from build123d import *
from build123d.topology import SkipClean

# Parameters (mm, degrees)
SKETCH1_W            = 10
SKETCH1_H            = 10
BOSS_EXTRUDE1_DEPTH  = 4.9
CHAMFER1_SIZE        = 1
BOSS_EXTRUDE2_DEPTH  = 16
BOSS_EXTRUDE3_DEPTH  = 10
BOSS_EXTRUDE4_DEPTH  = 13
CHAMFER2_SIZE        = 12
BOSS_EXTRUDE5_DEPTH  = 30
CUT_EXTRUDE2_REACH   = 128.798
CUT_EXTRUDE1_START   = -15
CUT_EXTRUDE1_DEPTH   = 15
M3_CLEARANCE_HOLE1_D = 3.6
SKETCH11_W           = 1.8
SKETCH11_H           = 4.9
CHAMFER3_SIZE        = 9
CHAMFER3_SIZE_2      = 7.926193673
SKETCH14_R           = 1.8
BOSS_EXTRUDE6_DEPTH  = 12
M3_CLEARANCE_HOLE3_D = 3.6
SKETCH19_W           = 25
SKETCH19_H           = 20
CUT_EXTRUDE3_DEPTH   = 3.062116


# Read off the part's stored shape, not the designer's step: Cut-Extrude1
# Some blends are built 0.0001 mm under size
with BuildPart() as part:
    # Sketch1 → Boss-Extrude1 (new body)
    with BuildSketch(Plane(origin=(0, 0, 0), x_dir=(1, 0, 0), z_dir=(0, 1, 0))):
        with Locations((-5, 5)):
            Rectangle(SKETCH1_W, SKETCH1_H)
    extrude(amount=BOSS_EXTRUDE1_DEPTH)

    # Chamfer1
    chamfer1_edges = [part.edges().sort_by_distance(p)[0] for p in [
        (-10, 0, -5),
    ]]
    chamfer(chamfer1_edges, length=CHAMFER1_SIZE)

    # Sketch2 → Boss-Extrude2 (add)
    with BuildSketch(Plane(origin=(0, 0, -10), x_dir=(-1, 0, 0), z_dir=(0, 0, -1))):
        Polygon((-49.9, -10.1), (-48.419662682, -10.1), (-46.146212445, -7.037883957), (1.467233005, 0), (9, 0), (10, 1), (10, 4.9), (0, 4.9), (-45.9, -1.884614526), (-45.9, 4.9), (-95.9, 4.9), (-95.9, 1.9), (-49.9, 1.9), align=None)
    extrude(amount=BOSS_EXTRUDE2_DEPTH)

    # Sketch2<4> → Boss-Extrude3 (add)
    with BuildSketch(Plane(origin=(0, 0, -10), x_dir=(-1, 0, 0), z_dir=(0, 0, -1))):
        Polygon((-49.9, -10.1), (-48.419662682, -10.1), (-46.146212445, -7.037883957), (1.467233005, 0), (0, 0), (0, 4.9), (-45.9, -1.884614526), (-45.9, 4.9), (-95.9, 4.9), (-95.9, 1.9), (-49.9, 1.9), align=None)
    extrude(amount=-BOSS_EXTRUDE3_DEPTH)

    # Sketch3 → Boss-Extrude4 (add)
    with BuildSketch(Plane(origin=(0, 0, -26), x_dir=(-1, 0, 0), z_dir=(0, 0, -1))):
        Polygon((-95.9, 1.9), (-95.9, -10.1), (-49.9, -10.1), (-48.419662682, -10.1), (-46.146212445, -7.037883957), (1.467233005, 0), (9, 0), (10, 1), (10, 4.9), (0, 4.9), (-45.9, -1.884614526), (-45.9, 4.9), (-95.9, 4.9), align=None)
    extrude(amount=BOSS_EXTRUDE4_DEPTH)

    # Chamfer2
    chamfer2_edges = [part.edges().sort_by_distance(p)[0] for p in [
        (72.9, -10.1, -26),
    ]]
    chamfer(chamfer2_edges, length=CHAMFER2_SIZE - 0.0001)  # a hair under: the kernel refuses the full size

    # Sketch4 → Boss-Extrude5 (add)
    with BuildSketch(Plane(origin=(0, 0, -39), x_dir=(-1, 0, 0), z_dir=(0, 0, -1))):
        Polygon((-95.9, 4.9), (-95.9, -10.1), (-48.419662682, -10.1), (-46.146212445, -7.037883957), (1.467233005, 0), (9, 0), (10, 1), (10, 4.9), (0, 4.9), (-45.9, -1.884614526), (-45.9, 4.9), align=None)
    extrude(amount=BOSS_EXTRUDE5_DEPTH)

    # Sketch15 → Cut-Extrude2 (cut, up to next)
    with BuildSketch(Plane(origin=(95.9, 0, 0), x_dir=(0, 0, -1), z_dir=(1, 0, 0)), mode=Mode.PRIVATE) as cut_extrude2_sk1:
        Polygon((69, -1.884614526), (35.441468776, -1.884614526), (28.656854249, 4.9), (69, 4.9), align=None)
    cut_extrude2_tool1 = extrude(cut_extrude2_sk1.sketch, amount=-CUT_EXTRUDE2_REACH, mode=Mode.PRIVATE) & part.part
    add(cut_extrude2_tool1.solids().sort_by_distance((95.9, 1.611504, -50.472675))[0], mode=Mode.SUBTRACT)

    # Cut-Extrude1 outline → Cut-Extrude1 (cut)
    with BuildSketch(Plane(origin=(0, 4.9, 0), x_dir=(1, 0, 0), z_dir=(0, 1, 0)).offset(CUT_EXTRUDE1_START)):
        with BuildLine():
            ThreePointArc((-10, 41.287361933), (51.179168383, 47.220256879), (90.528084846, 0))
            Line((90.528084846, 0), (95.9, 0))
            Line((95.9, 0), (95.9, 69))
            Line((95.9, 69), (-10, 69))
            Line((-10, 69), (-10, 41.287361933))
        make_face()
    extrude(amount=CUT_EXTRUDE1_DEPTH, mode=Mode.SUBTRACT)

    # M3 Clearance Hole1 (through all)
    with Locations(Plane(origin=(0, 1.9, 0), x_dir=(-1, 0, 0), z_dir=(0, -1, 0))):
        with Locations((-81.2, 7), (-54.2, 7)):
            Hole(M3_CLEARANCE_HOLE1_D / 2)

    # Sketch11 → M3 Clearance Hole2 (revolve, cut)
    with BuildSketch(Plane(origin=(-1.8, 0, -7), x_dir=(0, 0, -1), z_dir=(1, 0, 0))):
        with Locations((0.9, 2.45)):
            Rectangle(SKETCH11_W, SKETCH11_H)
    revolve(axis=Axis((-1.8, -6.35, -7), (0, 1, 0)), mode=Mode.SUBTRACT)

    # Chamfer3
    # the kernel refuses this chamfer: 9, 7.926193673 mm, written as the material it adds along each edge
    with BuildSketch(Plane(origin=(45.9, -1.884614526, -35.441468776), x_dir=(-0.9928980217571691, 0.11896856051369163, 0), z_dir=(0, 0, 1))) as chamfer3_piece_1_section:
        Polygon((CHAMFER3_SIZE * 0.999621916911, -CHAMFER3_SIZE * 0.0274958766106), (CHAMFER3_SIZE_2 * 0.118968560518, -CHAMFER3_SIZE_2 * 0.992898021792), (0, 0), align=None)
    chamfer3_piece_1 = extrude(amount=35.441468776, mode=Mode.PRIVATE)
    chamfer3_piece_1 = split(chamfer3_piece_1, bisect_by=Plane(origin=(42.836377778, 4.9, -16.273200987), z_dir=(0, -1, 0)), keep=Keep.TOP, mode=Mode.PRIVATE)
    chamfer3_piece_1 = split(chamfer3_piece_1, bisect_by=Plane(origin=(42.836377778, 9.147052769, -24.40980148), z_dir=(6.542051911182403e-15, -0.7071067811865479, 0.7071067811865472)), keep=Keep.TOP, mode=Mode.PRIVATE)
    add(chamfer3_piece_1)

    # Sketch12 → Cut-Revolve1 (revolve, cut)
    with BuildSketch(Plane.XY.offset(-25)):
        Polygon((0, -0.5), (22, -0.5), (92, -7.331568331), (90.828874, -19.331568331), (0, -10.467230343), align=None)
    revolve(axis=Axis((90.828874, -19.331568331, -25), (-0.9952714730097288, 0.09713235821828223, 0)), mode=Mode.SUBTRACT)

    # Sketch14 → Boss-Extrude6 (add)
    # profile 1 of 2: a face of its own
    with SkipClean():  # the faces are left unmerged after this step: merging them gives an invalid solid
        with BuildSketch(Plane.XZ.offset(-1.9)):
            with BuildLine():
                Line((83.95, -12.5), (86.547763007, -12.5))
                ThreePointArc((86.547763007, -12.5), (88.850452987, -6.3495173), (90.528084846, 0))
                Line((90.528084846, 0), (79.15, 0))
                Line((79.15, 0), (79.15, -9.7))
                Line((79.15, -9.7), (83.95, -9.7))
                Line((83.95, -9.7), (83.95, -12.5))
            make_face()
            with Locations(Location((81.2, -7, 0), (0, 0, 270))):
                Circle(SKETCH14_R, mode=Mode.SUBTRACT)
        # profile 2 of 2: a face of its own
        with BuildSketch(Plane.XZ.offset(-1.9)):
            Polygon((49.9, 0), (49.9, -12.5), (51.45, -12.5), (51.45, -9.7), (56.25, -9.7), (56.25, 0), align=None)
            with Locations(Location((54.2, -7, 0), (0, 0, 270))):
                Circle(SKETCH14_R, mode=Mode.SUBTRACT)
        extrude(amount=BOSS_EXTRUDE6_DEPTH)
    add(part.part.scale(1), mode=Mode.REPLACE)  # the faces are merged on a copy

    # M3 Clearance Hole3 (through all)
    with Locations(Plane(origin=(0, 4.9, 0), x_dir=(1, 0, 0), z_dir=(0, 1, 0))):
        with Locations((-1.8, 7)):
            Hole(M3_CLEARANCE_HOLE3_D / 2)

    # Sketch19 → Cut-Extrude3 (cut)
    with BuildSketch(Plane.XZ.offset(10.1)):
        with Locations((58.646212445, -40)):
            Rectangle(SKETCH19_W, SKETCH19_H)
    extrude(amount=-CUT_EXTRUDE3_DEPTH, mode=Mode.SUBTRACT)


solid = part.part
Build history of the part. All positions in model axes, mm. A direction names the side the tool comes from. Round coordinates to 2 decimals unless told otherwise and drop trailing zeros. Write each loop counter-clockwise with the first axis right and the second up, starting at its lowest first coordinate (ties: lowest second). Pieces come first, ordered by that corner, then holes. Notation, with made-up numbers: (-40, -3) - (0, -3) arc R32 ccw to (0, 29) - close; hole circle Ø8 at (67.25, 72.25). An arc over 180 degrees is marked (long way). One line per question, with ' | ' between items.
1. Band-saw the part on A-A, the plane y = 3.5. Write the cut outline in (x, z), and give its area (3 significant figures).
Results are:
outline: (-10, -41.29) arc R65.75 ccw to (9.47, -49.99) - (9.47, 0) - (-10, 0) - close; (42.48, -30.06) - (75.36, -30.06) arc R65.75 ccw to (90.53, 0) - (42.48, 0) - close; hole circle Ø3.6 at (-1.8, -7); hole circle Ø3.6 at (54.2, -7); hole circle Ø3.6 at (81.2, -7) | area: 2,140 mm^2
2. Tool access for faces 4 (the face through (82, -4, -9.7)), 5 (the face through (49.9, -3, -19)), 6 (the face through (79.15, -4, -5)), 7 (the face through (51.45, -4, -11)), 8 (the face through (-5, 0, -23)): list every direction of +Z, -Z, +X, -X, +Y, -Y with a clear straight run to the whole face (end or side of a thin tool).
Results are:
face 4: -Z, -Y | face 5: +X, -Y | face 6: +Z, -Z, -Y | face 7: -Y | face 8: +Z, -Z, -X, -Y
3. Drop flat-ended pins along their axis: pin 1 Ø1.5 at (y, z) = (-5.5, -37.5) entering from +X; pin 2 Ø1.7 at (x, y) = (51, -4.5) entering from -Z; pin 3 Ø8 at (x, y) = (70, -3.5) entering from +Z; pin 4 Ø3 at (x, z) = (81.2, -7) entering from +Y. Give the stop position or say it passes through.
Results are:
pin 1: x = 68.48 | pin 2: z = -47.63 | pin 3: z = -27.4 | pin 4: through
4. Mould opens along Z. For faces 1 (the face through (85, -4, -12.5)), 2 (the face through (68, 4.9, -14)), 3 (the face through (54, -4, -9.7)) say: released by +Z, released by -Z, zero draft, split by the parting line, or undercut.
Results are:
face 1: released by -Z | face 2: zero draft | face 3: undercut
5. Drill centre lines: line 1 along Z through (x, y) = (81.2, -5.25); line 2 along Z through (x, y) = (55, -4.75); line 3 along Z through (x, y) = (54.2, -1). Where is each one in solid material? Low to high. Write a range as from..to.
Results are:
line 1: -9.7..-8.8, -5.2..0 | line 2: -45.51..-32.65, -9.7..-8.61, -5.39..0 | line 3: -34.56..-28.9, -9.7..-8.8, -5.2..0
6. Band-saw the part on C-C, the plane y = -5.5. Give the number of separate pieces and of enclosed holes in the cut face, and give its area (3 significant figures).
Results are:
separate pieces: 3 | enclosed holes: 2 | area: 819 mm^2
